Part print with two shaded views. Sizes in mm from the minimum x, y, z corner. Give positions to 0.01 mm unless a question says otherwise; leave off trailing zeros. Write each loop counter-clockwise with the first axis right and the second up, starting at its lowest first coordinate (ties: lowest second). Pieces come first, ordered by that corner, then holes.
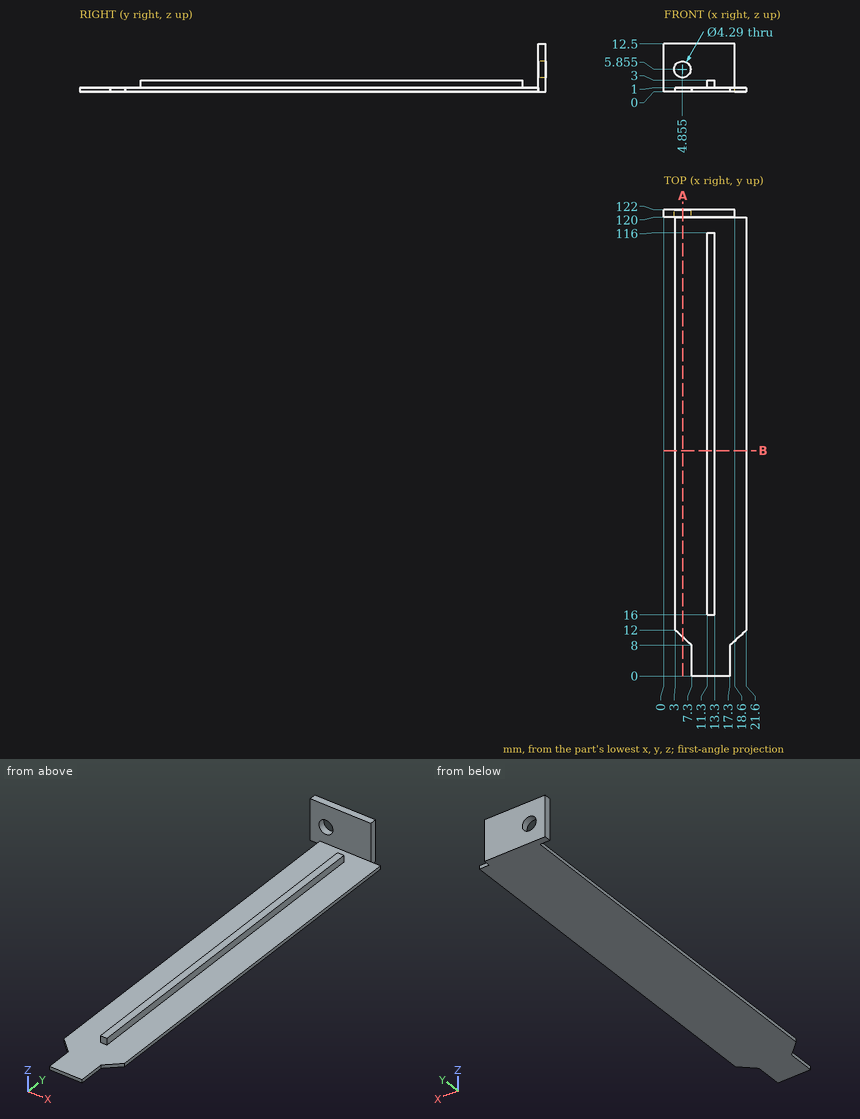
1) Saw through at B-B (y = 59). Write the cut outline in (x, z), and give its area (3 significant figures).
Check result:
outline: (3, 0) - (21.6, 0) - (21.6, 1) - (13.3, 1) - (13.3, 3) - (11.3, 3) - (11.3, 1) - (3, 1) - close
area: 22.6 mm2
2) Drill centre lines: L1, parallel to X at y = 23.5, z = 1.5; L2, parallel to Z at x = 6.5, y = 23; L3, parallel to Y at x = 14, z = 10. Where is each one in solid material? Low to high.
Check result:
L1: x = 11.3 to 13.3
L2: z = 0 to 1
L3: y = 120 to 122
3) Flat gauge pins, fed straight in: P1, Ø0.5, axis at x = 20, z = 0.5, coming from the +Y side; P2, Ø3, axis at x = 14, z = 4.5, coming from the -Y side; P3, Ø1, axis at x = 12.5, y = 81.5, coming from the +Z side. Where does each tip first touch, or does it go through?
Check result:
P1: stops at y = 120
P2: stops at y = 120
P3: stops at z = 3
4) Saw through at A-A (x = 5). Write the cut outline in (y, z), and give its area (3 significant figures).
Check result:
outline: (10.14, 0) - (122, 0) - (122, 3.71) - (120, 3.71) - (120, 1) - (10.14, 1) - close; (120, 8) - (122, 8) - (122, 12.5) - (120, 12.5) - close
area: 126 mm2
